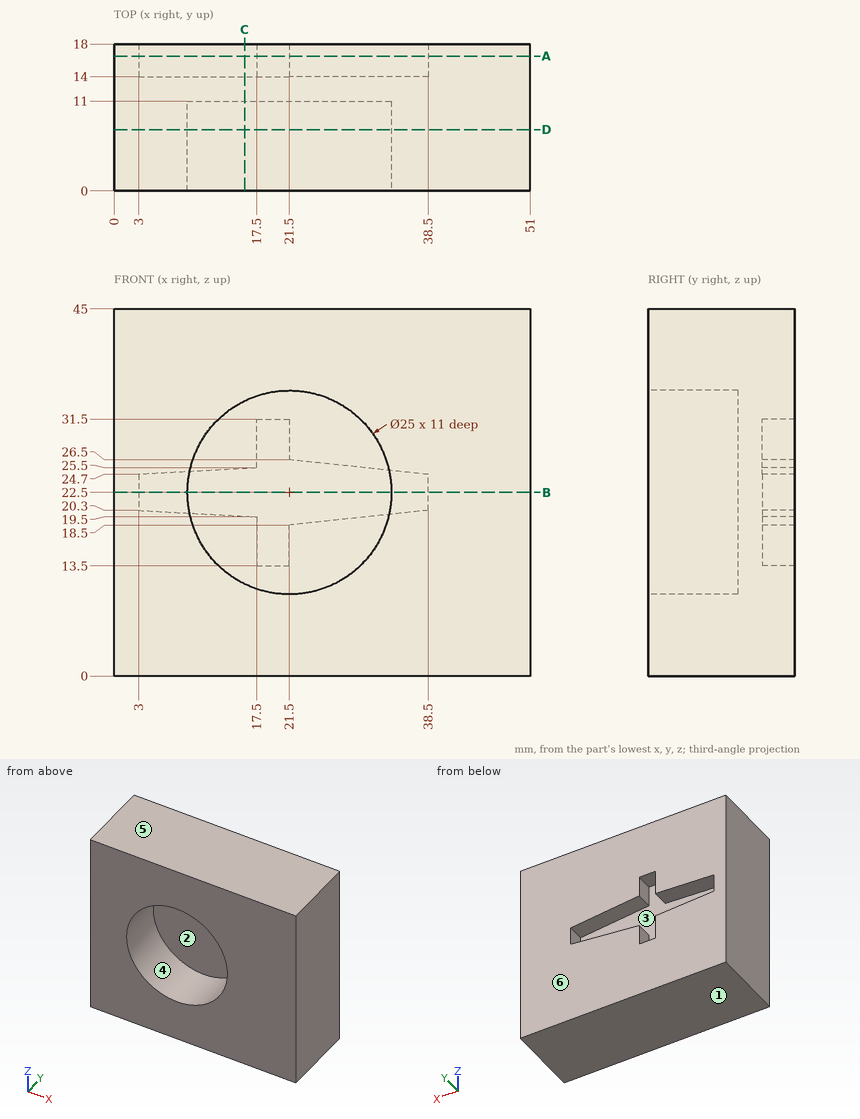
Answer from the drawing. Dimensions are ordinates in mm from the lowest x, y and z of the part. A direction names the side the tool comes from. Round coordinates to 2 decimals unless told otherwise and drop trailing zeros. Write each loop counter-clockwise with the first axis right and the second up, starting at its lowest first coordinate (ties: lowest second). Pieces come first, ordered by that corner, then holes. Notation, with made-up numbers: M 34,3.5 L 40,3.5 A4 ccw 40,9.5 Z; hole C 52.5,53 d10. An arc over 180 degrees is marked long. Write each question's results on one line, items separated by ' | '. Start each with the question number.
Item 1: Find section C-C on x = 16. Write down the section's boundary in (y, z), and give its area (3 significant figures).
Item 2: Find section D-D on y = 7.5. Write down the section's boundary in (x, z).
Item 3: Find section B-B on z = 22.5. Write down the section's boundary in (x, y).
Item 4: Which of the six approach directions +Z, -Z, +X, -X, +Y, -Y give full straight-line access (tool end or side, diameter ignored) to the marked faces 1, 2 and 3?
Item 5: The mould has two halves that part along Z. Classify the marked faces 4, 5 and 6: +Z half, -Z half, draft (parallel to the pull), parting line (faces both ways), or undercut.
Item 6: Straight lines are drawn through the part: probe 1 along Z at (x, y) = (21.5, 3); probe 2 along Y at (x, z) = (22, 31); probe 3 along Y at (x, z) = (19, 16.5). For each, find the intervals that lie inside material, in ascending order.
Item 7: Find section A-A on y = 16.5. Write down the section's boundary in (x, z).
Answer block:
1) outline: M 0,0 L 18,0 L 18,19.58 L 14,19.58 L 14,25.42 L 18,25.42 L 18,45 L 0,45 L 0,33.72 L 11,33.72 L 11,11.28 L 0,11.28 Z | area: 540 mm²
2) outline: M 0,0 L 51,0 L 51,45 L 0,45 Z; hole C 21.5,22.5 d25
3) outline: M 0,0 L 9,0 L 9,11 L 34,11 L 34,0 L 51,0 L 51,18 L 38.5,18 L 38.5,14 L 3,14 L 3,18 L 0,18 Z
4) face 1: -Z, +X, -X, +Y, -Y | face 2: -Y | face 3: +Y
5) face 4: undercut | face 5: +Z half | face 6: draft
6) probe 1: z = 0 to 10, 35 to 45 | probe 2: y = 11 to 18 | probe 3: y = 11 to 14
7) outline: M 0,0 L 51,0 L 51,45 L 0,45 Z; hole M 3,20.3 L 17.5,19.5 L 17.5,13.5 L 21.5,13.5 L 21.5,18.5 L 38.5,20.3 L 38.5,24.7 L 21.5,26.5 L 21.5,31.5 L 17.5,31.5 L 17.5,25.5 L 3,24.7 Z
